from build123d import *

# Parameters (mm, degrees)
SKETCH1_R           = 9.525
BOSS_EXTRUDE1_DEPTH = 400
SKETCH2_W           = 30
SKETCH2_H           = 35
BOSS_EXTRUDE2_DEPTH = 10
FILLET1_R           = 3


with BuildPart() as part:
    # Sketch1 → Boss-Extrude1 (new body)
    with BuildSketch(Plane.XY):
        Circle(SKETCH1_R)
    extrude(amount=BOSS_EXTRUDE1_DEPTH)

    # Sketch2 → Boss-Extrude2 (add)
    with BuildSketch(Plane.XY.offset(400)):
        with Locations((0, 7.5)):
            Rectangle(SKETCH2_W, SKETCH2_H)
    extrude(amount=BOSS_EXTRUDE2_DEPTH)

    # Fillet1
    fillet1_edges = [part.edges().sort_by_distance(p)[0] for p in [
        (-15, 25, 405),
        (-15, -10, 405),
        (15, -10, 405),
        (15, 25, 405),
    ]]
    fillet(fillet1_edges, radius=FILLET1_R)


solid = part.part
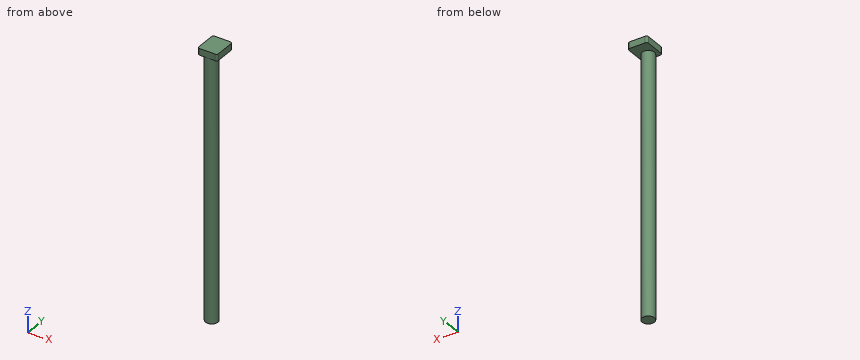
The listing builds one solid part. Answer for the finished solid, in the listing's coordinates (mm). Round coordinates to 2 decimals unless told otherwise and drop trailing zeros. Write each loop counter-clockwise with the first axis right and the second up, starting at its lowest first coordinate (ties: lowest second). Pieces come first, ordered by that corner, then holes. Notation, with made-up numbers: (41.5, -0.75) - (63.5, -0.75) arc R32 cw to (63.5, 36.25) - close; hole circle Ø2 at (-8, -32). An arc over 180 degrees is marked (long way). Use one line per item in the form item = value. Start each with the question number.
Item 1: A cutting plane is placed at A-A (x = 0). Write down the section's boundary in (y, z) (3 decimals), plus the area to 3 significant figures.
Item 2: Flat-ended cylindrical pins translate along their axes: pin 1 Ø3 at (y, z) = (6.5, 226.5) entering from -X; pin 2 Ø6 at (x, z) = (-5, 190.5) entering from +Y; pin 3 Ø10 at (x, z) = (-4.5, 182) entering from +Y (3 decimals). Find the tip coordinate at first contact, or state that the pin passes through.
Item 3: Find the intervals of material crossed by line 1 (Z direction, x = 12.75, y = 23); line 2 (Y direction, x = 1, z = 337.5), in increasing order. Write a range as [from, to].
Item 4: A cutting plane is placed at C-C (z = 96). Write down the section's boundary in (x, y) (3 decimals).
Item 5: A cutting plane is placed at B-B (y = 0). Write down the section's boundary in (x, z) (3 decimals).
The answers:
q1.outline = (-10, 400) - (-9.525, 400) - (-9.525, 0) - (9.525, 0) - (9.525, 400) - (25, 400) - (25, 410) - (-10, 410) - close
q1.area = 7,970 mm^2
q2.pin_1 = -8.11
q2.pin_2 = 9.31
q2.pin_3 = 9.525
q3.line_1 = [400, 410]
q3.line_2 = [-9.47, 9.47]
q4.outline = circle Ø19.05 at (0, 0)
q5.outline = (-15, 400) - (-9.525, 400) - (-9.525, 0) - (9.525, 0) - (9.525, 400) - (15, 400) - (15, 410) - (-15, 410) - close
